Here's how the part is built. I have some questions about the finished solid (model axes, mm). Face numbers are marked on the shaded views. A direction names the side the tool comes from. Round coordinates to 2 decimals unless told otherwise and drop trailing zeros. Write each loop counter-clockwise with the first axis right and the second up, starting at its lowest first coordinate (ties: lowest second). Pieces come first, ordered by that corner, then holes. Notation, with made-up numbers: (-11, -5) - (45, -5) arc R24 ccw to (45, 15) - close; hole circle Ø4 at (-29.5, -20.5). An arc over 180 degrees is marked (long way). One line per item, written item: value. Start each with the question number.
Item 1: For P1, Ø8, axis at x = 79, z = 53, coming from the -Y side; P2, Ø2, axis at x = 65, z = 61.5, coming from the -Y side; P3, Ø2, axis at x = 72, z = 62.5, coming from the -Y side, each with a flat end and sliding along its axis, tell me the tip position at first contact or that it passes through.
Item 2: Thinking about a two-plate mould opening in Z: for the marked faces 3, 4 and 5, which applies, released by +Z, released by -Z, zero draft, split by the parting line, or undercut?
Item 3: For the marked faces 1 and 2, which set-ups out of +Z, -Z, +X, -X, +Y, -Y let a thin tool reach every point of the face, with its end or its side?
Item 4: Imagine slicing it at A-A, the plane x = 58.5. Please give me the cut outline in (y, z), then the cut area to 3 significant figures.
Item 5: If I drill on line 1 (X direction, y = 29.5, z = 51.5); line 2 (Z direction, x = 103.5, y = 33); line 3 (Y direction, x = 100, z = 67), over which ranges is the centre line in solid material (lowest first)?
Item 6: Imagine slicing it at B-B, the plane x = 80.5. Please give me the cut outline in (y, z).
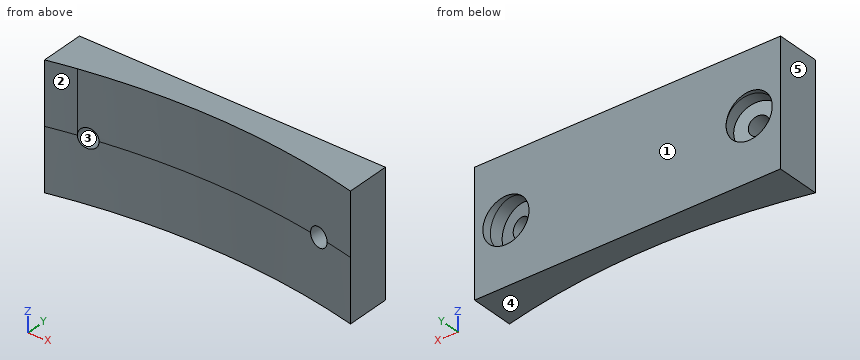
Autodesk Inventor part; units mm, degrees
ref_plane "YZ Plane" through (0, 0, 0) normal (1, 0, 0) x (0, 1, 0)
ref_plane "XZ Plane" through (0, 0, 0) normal (0, 1, 0) x (-1, 0, 0)
ref_plane "XY Plane" through (0, 0, 0) normal (0, 0, 1) x (1, 0, 0)
sketch "Sketch3" plane through (0, 0, 0) normal (0, 0, 1) x (1, 0, 0)
  line L0 (11.505, 42.3202) -> (113.105, 42.3202)
  line L1 (113.105, 42.3202) -> (113.105, 16.9202)
  line L2 (113.105, 16.9202) -> (11.505, 16.9202)
  line L3 (11.505, 16.9202) -> (11.505, 42.3202)
  point P0 (0, 0)
  dimension "d11" = 101.6
  dimension "d12" = 25.4
extrude "Extrusion1" add sketch "Sketch3" along normal blind 50.8
sketch "Sketch4" plane through (0, 0, 50.8) normal (0, 0, 1) x (1, 0, 0)
  line L0 (11.505, 16.9202) -> (113.105, 16.9202)
  line L1 (62.305, 23.2702) -> (62.305, 26.3182)
  line L2 (97.738, 23.2702) -> (26.872, 23.2702)
  circle A0 centre (62.305, -181.1601) radius 207.4783
  point P0 (0, 0)
extrude "Extrusion2" cut sketch "Sketch4" against normal blind 50.8
sketch "Sketch6" plane through (0, 0, 50.8) normal (0, 0, 1) x (1, 0, 0)
  arc A0 (113.105, 20.003) -> (11.505, 20.003) centre (62.305, -181.1601) ccw
  line L0 (62.305, 26.3182) -> (62.305, 23.2702)
  line L1 (62.305, 23.2702) -> (26.872, 23.2702)
  line L2 (26.872, 23.2702) -> (97.738, 23.2702)
  arc A1 (97.738, 23.2702) -> (26.872, 23.2702) centre (62.305, -181.1601) ccw
  line L3 (26.872, 23.2702) -> (29.8127, 23.7797)
  line L4 (26.872, 23.2702) -> (29.8565, 23.2702) construction
  line L5 (29.8127, 23.7797) -> (28.7286, 30.0365)
  line L6 (28.7286, 30.0365) -> (32.6703, 30.7195)
  line L7 (32.6703, 30.7195) -> (32.0199, 34.4735)
  line L8 (26.872, 23.2702) -> (22.5356, 48.2973)
  line L9 (26.872, 23.2702) -> (52.272, 23.2702) construction
  line L10 (22.5356, 48.2973) -> (29.418, 49.4898)
  line L11 (29.418, 49.4898) -> (32.0199, 34.4735)
  line L12 (29.8127, 23.7797) -> (29.9804, 22.8117)
  line L13 (29.9804, 22.8117) -> (27.0397, 22.3022)
  line L14 (27.0397, 22.3022) -> (26.872, 23.2702)
  point P0 (0, 0)
  dimension "d39" = 3.048
  dimension "d40" = 35.433
  dimension "d41" = 2.9845
  dimension "d42" = 9.83
  dimension "d43" = 6.35
  dimension "d44" = 90
  dimension "d45" = 4.0005
  dimension "d46" = 90
  dimension "d47" = 3.81
  dimension "d48" = 25.4
  dimension "d49" = 99.83
revolve "Revolution1" cut sketch "Sketch6" angle 360 about axis through (26.872, 23.2702, 50.8) along (-0.1707254, 0.9853186, 0) contours L12 L1 A0 | A0 L3 L12 | L12 L13 L14 L1 | L8 L10 L11 L7 L6 L5 L3
ref_plane "Work Plane2" through (62.305, 42.3202, 50.8) normal (1, 0, 0) x (0, 0, -1)
mirror "Mirror1" about plane through (62.305, 42.3202, 50.8) normal (1, 0, 0) of "Revolution1"
sketch "Sketch7" plane through (0, 0, 50.8) normal (0, 0, 1) x (1, 0, 0)
  line L0 (18.9054, 28.3344) -> (16.4821, 42.3202)
  line L1 (18.9054, 28.3344) -> (18.255, 32.0885)
  line L2 (18.255, 32.0885) -> (32.0199, 34.4735)
  line L3 (32.0199, 34.4735) -> (32.6703, 30.7195)
  line L4 (32.0199, 34.4735) -> (113.105, 34.4735)
  line L5 (113.105, 20.003) -> (113.105, 42.3202)
  line L6 (16.4821, 42.3202) -> (11.505, 42.3202)
  line L7 (113.105, 34.4735) -> (11.505, 34.4735)
  line L8 (11.505, 34.4735) -> (11.505, 42.3202)
  line L9 (11.505, 42.3202) -> (113.105, 42.3202)
  line L10 (113.105, 42.3202) -> (113.105, 34.4735)
  point P0 (0, 0)
  dimension "d52" = 3.81
  dimension "d53" = 13.97
  dimension "d54" = 90
extrude "Extrusion3" cut sketch "Sketch7" against normal blind 50.8 contours L7 L8 L6 L0 | L0 L9 L5 L4 L7
sketch "Sketch8" plane through (0, 0, 50.8) normal (0, 0, 1) x (1, 0, 0)
  line L0 (18.9054, 28.3344) -> (17.8417, 34.4735)
  line L1 (17.8417, 34.4735) -> (15.3017, 34.4735)
  line L2 (11.505, 34.4735) -> (113.105, 34.4735)
  line L3 (15.3017, 34.4735) -> (15.3017, 16.7671)
  line L4 (15.3017, 16.7671) -> (7.6342, 16.7671)
  line L5 (7.6342, 16.7671) -> (7.6342, 34.4735)
  line L6 (7.6342, 34.4735) -> (15.3017, 34.4735)
  line L7 (62.305, 34.4735) -> (62.305, 19.3718)
  line L8 (109.3083, 34.4735) -> (109.3083, 16.7671)
  line L9 (109.3083, 16.7671) -> (116.9758, 16.7671)
  line L10 (116.9758, 16.7671) -> (116.9758, 34.4735)
  line L11 (116.9758, 34.4735) -> (109.3083, 34.4735)
  point P0 (0, 0)
  dimension "d57" = 2.54
extrude "Extrusion4" cut sketch "Sketch8" against normal blind 50.8
sketch "Sketch9" plane through (0, 0, 0) normal (0, 0, -1) x (-1, 0, 0)
  line L0 (-123.5208, 45.9759) -> (-4.4224, 45.9759)
  line L1 (-4.4224, 45.9759) -> (-4.4224, 6.2764)
  line L2 (-4.4224, 6.2764) -> (-123.5208, 6.2764)
  line L3 (-123.5208, 6.2764) -> (-123.5208, 45.9759)
  point P0 (0, 0)
extrude "Extrusion5" cut sketch "Sketch9" against normal blind 31.75
sketch "Sketch10" plane through (0, 0, 50.8) normal (0, 0, 1) x (1, 0, 0)
  arc A0 (23.935, 22.7393) -> (15.3017, 20.9239) centre (62.305, -181.1601) ccw
  line L0 (15.3017, 34.4735) -> (15.3017, 20.9239)
  line L1 (15.3017, 20.9239) -> (15.3017, 34.4735)
  line L2 (109.3083, 20.9239) -> (109.3083, 34.4735)
  line L3 (15.3017, 34.4735) -> (109.3083, 34.4735)
  line L4 (109.3083, 34.4735) -> (109.3083, 20.9239)
  arc A1 (109.3083, 20.9239) -> (15.3017, 20.9239) centre (62.305, -181.1601) ccw
  point P0 (0, 0)
  point P1 (23.935, 22.7393)
extrude "Extrusion6" add sketch "Sketch10" along normal blind 19.05
mirror "Mirror5" about plane through (62.305, 27.6987, 50.8) normal (0, 0, -1) of "Revolution1", "Mirror1"
properties part number "MountPlateV1"
Values follow:
1. P1: stops at y = 25.28
1. P2: stops at y = 26.29
1. P3: stops at y = 26.04
2. face 3: undercut
2. face 4: released by -Z
2. face 5: zero draft
3. face 1: +Z, -Z, +X, -X, +Y
3. face 2: +Z, -Z, -Y
4. outline: (26.28, 31.75) - (34.47, 31.75) - (34.47, 69.85) - (26.28, 69.85) - close
4. area: 312 mm^2
5. line 1: x = 15.3 to 18.74, 28.74 to 95.87, 105.87 to 109.31
5. line 2: z = 31.75 to 45.09, 56.51 to 69.85
5. line 3: y = 22.87 to 34.47
6. outline: (25.52, 31.75) - (34.47, 31.75) - (34.47, 69.85) - (25.52, 69.85) - close
